```python
from build123d import *

# Parameters (mm, degrees)
SKETCH_1_W      = 10
SKETCH_1_H      = 40
SKETCH_1_W_2    = 5
SKETCH_1_H_2    = 10
EXTRUDE_1_DEPTH = 40
FILLET_2_R      = 5
FILLET_3_R      = 2.5
FILLET_4_R      = 2.5
FILLET_6_R      = 2


with BuildPart() as part:
    # 草圖1 → 填料-伸長1 (new body)
    with BuildSketch(Plane.XY):
        with Locations((-34.732391425, 13.59375)):
            Rectangle(SKETCH_1_W, SKETCH_1_H)
        Polygon((-29.732391425, -6.40625), (-39.732391425, -6.40625), (-39.732391425, -16.40625), (35.267608575, -16.40625), (35.267608575, -6.40625), (30.267608575, -6.40625), (-14.732391425, -6.40625), (-19.732391425, -6.40625), align=None)
        with Locations((-17.232391425, -1.40625)):
            Rectangle(SKETCH_1_W_2, SKETCH_1_H_2)
        with Locations((32.767608575, -1.40625)):
            Rectangle(SKETCH_1_W_2, SKETCH_1_H_2)
    extrude(amount=EXTRUDE_1_DEPTH)

    # 圓角2
    fillet_2_edges = [part.edges().sort_by_distance(p)[0] for p in [
        (-29.732391425, 33.59375, 20),
    ]]
    fillet(fillet_2_edges, radius=FILLET_2_R)

    # 圓角3
    fillet_3_edges = [part.edges().sort_by_distance(p)[0] for p in [
        (-29.732391425, -6.40625, 20),
        (-19.732391425, -6.40625, 20),
    ]]
    fillet(fillet_3_edges, radius=FILLET_3_R)

    # 圓角4
    fillet_4_edges = [part.edges().sort_by_distance(p)[0] for p in [
        (30.267608575, -6.40625, 20),
        (30.267608575, 3.59375, 20),
        (35.267608575, 3.59375, 20),
        (-14.732391425, -6.40625, 20),
        (-14.732391425, 3.59375, 20),
        (-19.732391425, 3.59375, 20),
    ]]
    fillet(fillet_4_edges, radius=FILLET_4_R - 0.0001)  # a hair under: the kernel refuses the full size

    # 圓角6
    fillet_6_edges = [part.edges().sort_by_distance(p)[0] for p in [
        (-37.232391425, 33.59375, 40),
        (-37.232391425, 33.59375, 0),
        (-29.732391425, 12.34375, 0),
        (-31.196857519, 32.129283906, 0),
        (-29.732391425, 12.34375, 40),
        (-31.196857519, 32.129283906, 40),
        (-19.732391425, -1.4062, 0),
        (-19.732391425, -1.4062, 40),
        (-24.732391425, -6.40625, 0),
        (-24.732391425, -6.40625, 40),
        (-20.464624472, -5.674016953, 40),
        (-20.464624472, -5.674016953, 0),
        (-29.000158378, -5.674016953, 0),
        (-29.000158378, -5.674016953, 40),
        (30.267608575, -1.40625, 0),
        (30.267608575, -1.40625, 40),
        (7.767608575, -6.40625, 0),
        (7.767608575, -6.40625, 40),
        (-14.732391425, -1.40625, 0),
        (35.267608575, -7.6562, 0),
        (-19.000187668, 2.861546242, 0),
        (-15.464595183, 2.861546242, 0),
        (34.535404817, 2.861546242, 0),
        (30.999812332, 2.861546242, 0),
        (35.267608575, -7.6562, 40),
        (-14.732391425, -1.40625, 40),
        (-19.000187668, 2.861546242, 40),
        (-15.464595183, 2.861546242, 40),
        (34.535404817, 2.861546242, 40),
        (30.999812332, 2.861546242, 40),
        (29.535404817, -5.674046242, 40),
        (29.535404817, -5.674046242, 0),
        (-14.000187668, -5.674046242, 40),
        (-14.000187668, -5.674046242, 0),
    ]]
    fillet(fillet_6_edges, radius=FILLET_6_R)


solid = part.part
```
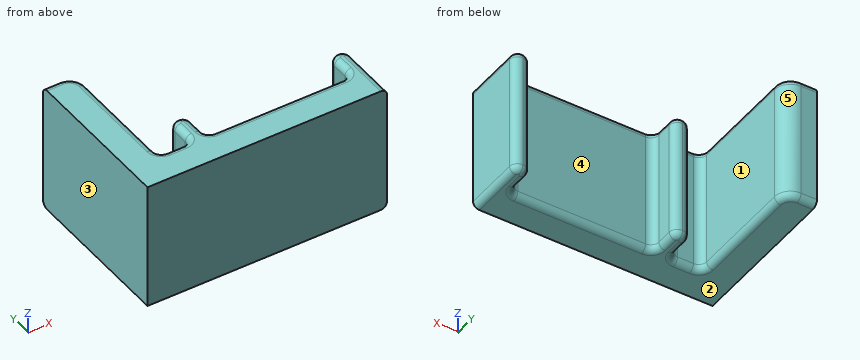
The model under review builds one solid part; all positions refer to its coordinate system, in mm. Face numbers are marked on the shaded views. A direction names the side the tool comes from. Give positions to 0.01 mm unless a question says otherwise; leave off trailing zeros. Write each loop counter-clockwise with the first axis right and the second up, starting at its lowest first coordinate (ties: lowest second). Pieces come first, ordered by that corner, then holes. Notation, with made-up numbers: M -25,-27 L -5,-27 A15 ccw -5,-22 Z; hole C -36.5,58.5 d3. An arc over 180 degrees is marked long. Write item = value, one per line. Start each with the question number.
Q1. We need section B-B (x = -2). State the section outline as (y, z) points.
Q2. Clearance check with a flat-ended pin moving along its axis: pin 1 (8 mm diameter, centred on x = 8.5, z = 5, fed in from +Y). State where the tip first meets the part, or that it passes through.
Q3. For line 1 (X direction, y = -3, z = 16.5); line 2 (X direction, y = 7.5, z = 26.5); line 3 (Y direction, x = 20, z = 12.5), list the stretches that pass through material, from the lowest coordinate up.
Q4. Mouldability with a two-part tool opening along X and no side actions: class the marked faces 1, 2 and 3 as released by +X, released by -X, zero draft, split by the parting line, or undercut.
Q5. We need section A-A (y = 16). State the section outline as (x, z) points, plus the area to 3 significant figures.
Q6. We need section D-D (y = 2.5). Give the number of separate pieces and of enclosed holes in the cut face, plus the area to 3 significant figures.
Q7. Machinability: for the marked faces 4 and 5, which of the approach directions +Z, -Z, +X, -X, +Y, -Y give a long, thin tool a straight path to every point of the face, cutting with its end or side? Answer none if there is none.
Result set:
q1.outline = M -16.41,0 L -8.41,0 A2 ccw -6.41,2 L -6.41,38 A2 ccw -8.41,40 L -16.41,40 Z
q2.pin_1 = -6.41
q3.line_1 = -39.73 to -29.73, -19.73 to -14.73, 30.27 to 35.27
q3.line_2 = -39.73 to -29.73
q3.line_3 = -16.41 to -6.41
q4.face_1 = undercut
q4.face_2 = zero draft
q4.face_3 = released by -X
q5.outline = M -39.73,0 L -31.73,0 A2 ccw -29.73,2 L -29.73,38 A2 ccw -31.73,40 L -39.73,40 Z
q5.area = 398 mm2
q6.separate_pieces = 3
q6.enclosed_holes = 0
q6.area = 719 mm2
q7.face_4 = +Z, -Z, +Y
q7.face_5 = +Z, -Z, +X, +Y
